CAD build for the part. Positions are in the model's coordinates, mm. Face numbers are marked on the shaded views. A direction names the side the tool comes from. Give positions to 0.01 mm unless a question says otherwise; leave off trailing zeros. Loops run counter-clockwise (first coordinate to the right, second up) from the corner with the lowest first, then second, coordinate; pieces in that order, holes last. Notation, with made-up numbers: M 7,-17 L 17,-17 A23 cw 17,-6 Z; hole C 22,70.25 d1. An arc over 180 degrees is marked long. Answer as CSV lines item,"result".
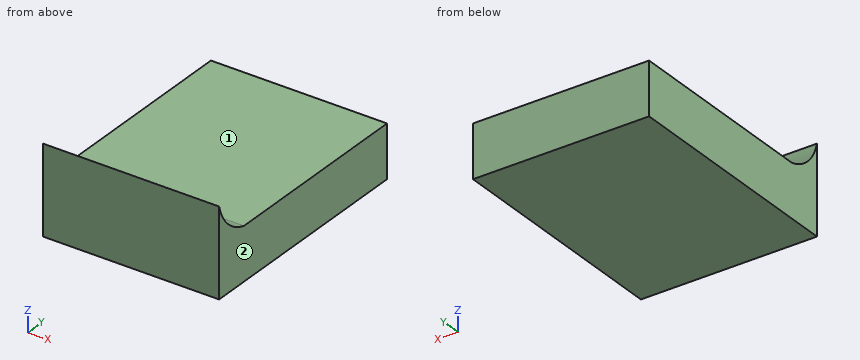
```python
from build123d import *

# Parameters (mm, degrees)
SKETCH_1_W      = 50
SKETCH_1_H      = 67.5
EXTRUDE_1_DEPTH = 15
EXTRUDE_2_DEPTH = 50


with BuildPart() as part:
    # 草图1 → 凸台-拉伸1 (new body)
    with BuildSketch(Plane.XY):
        Rectangle(SKETCH_1_W, SKETCH_1_H)
    extrude(amount=EXTRUDE_1_DEPTH)

    # 草图5 → 凸台-拉伸2 (add)
    with BuildSketch(Plane(origin=(25, 0, 0), x_dir=(0, 0, -1), z_dir=(1, 0, 0))):
        with BuildLine():
            Line((-15, -33.75), (-25, -33.75))
            ThreePointArc((-25, -33.75), (-18.575918968, -30.174081032), (-15, -23.75))
            Line((-15, -23.75), (-15, -33.75))
        make_face()
    extrude(amount=-EXTRUDE_2_DEPTH)


solid = part.part
```
Q1. Cut at C-C (y = -2.5). Write the cut outline in (x, z), and give its area (3 significant figures).
Solution:
outline,"M -25,0 L 25,0 L 25,15 L -25,15 Z"
area,"750 mm²"
Q2. Cut at B-B (z = 19). Write the cut outline in (x, y), and give its area (4 significant figures).
Solution:
outline,"M -25,-33.75 L 25,-33.75 L 25,-30.58 L -25,-30.58 Z"
area,"158.5 mm²"
Q3. Which spindle directions (+Z, -Z, +X, -X, +Y, -Y) get a long thin tool onto all of the face, cutting with end or side? Do the marked faces 1 and 2. Say none if no direction does.
Solution:
face 1,"+Z, +X, -X, +Y"
face 2,"+Z, -Z, +X, +Y, -Y"
Q4. Wall check: line 1 (Z direction, x = 22, y = -22); line 2 (Z direction, x = 5, y = -29.5); line 3 (Y direction, x = 0, z = 23.75). Give the ranges that are in metal, low to high. Write a range as [from, to].
Solution:
line 1,"z = [0, 15]"
line 2,"z = [0, 17.95]"
line 3,"y = [-33.75, -33.39]"
Q5. Cut at A-A (x = 3). Write the cut outline in (y, z).
Solution:
outline,"M -33.75,0 L 33.75,0 L 33.75,15 L -23.75,15 A13.42 cw -33.75,25 Z"
Q6. Pin check, flat tip, straight feed: P1, Ø1, axis at x = -3, y = 5.5, coming from the +Z side. Stop position of the tip, or through.
Solution:
P1,"stops at z = 15"
